Read the model definition and answer for the solid it produces. Units are mm, in the model's axes. A direction names the side the tool comes from. Give positions to 0.01 mm unless a question says otherwise; leave off trailing zeros. Write each loop counter-clockwise with the first axis right and the second up, starting at its lowest first coordinate (ties: lowest second). Pieces come first, ordered by that corner, then holes. Notation, with made-up numbers: (46, 41) -> (103, 41) arc R14 cw to (103, 52) -> close; hole circle Ø6 at (-2.75, 51). An arc over 180 degrees is marked (long way). Write item = value, one per line.
from build123d import *

# Parameters (mm, degrees)
CROQUIS1_W              = 240
CROQUIS1_H              = 260
SALIENTE_EXTRUIR1_DEPTH = 15
CROQUIS6_R              = 2.55
CORTAR_EXTRUIR3_DEPTH   = 178.552809046
CROQUIS7_R              = 5.5
CORTAR_EXTRUIR4_DEPTH   = 5
CROQUIS8_R              = 3.5
CORTAR_EXTRUIR5_DEPTH   = 178.552809046
CORTAR_EXTRUIR6_REACH   = 179.553
CROQUIS9_R              = 2.625
CROQUIS10_R             = 5.5
CORTAR_EXTRUIR7_DEPTH   = 5


with BuildPart() as part:
    # Croquis1 → Saliente-Extruir1 (new body)
    with BuildSketch(Plane(origin=(0, 0, 0), x_dir=(1, 0, 0), z_dir=(0, 1, 0))):
        Rectangle(CROQUIS1_W, CROQUIS1_H)
    extrude(amount=SALIENTE_EXTRUIR1_DEPTH)

    # Croquis6 → Cortar-Extruir3 (cut, through all)
    with BuildSketch(Plane.XZ):
        with Locations(Location((-45.5, -47.5, 0), (0, 0, 270))):
            Circle(CROQUIS6_R)
        with Locations(Location((-97.5, -47.5, 0), (0, 0, 270))):
            Circle(CROQUIS6_R)
        with Locations(Location((-97.5, 47.5, 0), (0, 0, 270))):
            Circle(CROQUIS6_R)
        with Locations(Location((-45.5, 47.5, 0), (0, 0, 270))):
            Circle(CROQUIS6_R)
        with Locations(Location((45.5, 47.5, 0), (0, 0, 270))):
            Circle(CROQUIS6_R)
        with Locations(Location((97.5, 47.5, 0), (0, 0, 270))):
            Circle(CROQUIS6_R)
        with Locations(Location((45.5, -47.5, 0), (0, 0, 270))):
            Circle(CROQUIS6_R)
        with Locations(Location((97.5, -47.5, 0), (0, 0, 270))):
            Circle(CROQUIS6_R)
    extrude(amount=-CORTAR_EXTRUIR3_DEPTH, mode=Mode.SUBTRACT)

    # Croquis7 → Cortar-Extruir4 (cut)
    with BuildSketch(Plane(origin=(0, 15, 0), x_dir=(1, 0, 0), z_dir=(0, 1, 0))):
        with Locations(Location((-97.5, 47.5, 0), (0, 0, 270))):
            Circle(CROQUIS7_R)
        with Locations(Location((-45.5, 47.5, 0), (0, 0, 270))):
            Circle(CROQUIS7_R)
        with Locations(Location((-97.5, -47.5, 0), (0, 0, 270))):
            Circle(CROQUIS7_R)
        with Locations(Location((-45.5, -47.5, 0), (0, 0, 270))):
            Circle(CROQUIS7_R)
        with Locations(Location((45.5, -47.5, 0), (0, 0, 270))):
            Circle(CROQUIS7_R)
        with Locations(Location((97.5, -47.5, 0), (0, 0, 270))):
            Circle(CROQUIS7_R)
        with Locations(Location((97.5, 47.5, 0), (0, 0, 270))):
            Circle(CROQUIS7_R)
        with Locations(Location((45.5, 47.5, 0), (0, 0, 270))):
            Circle(CROQUIS7_R)
    extrude(amount=-CORTAR_EXTRUIR4_DEPTH, mode=Mode.SUBTRACT)

    # Croquis8 → Cortar-Extruir5 (cut, through all)
    with BuildSketch(Plane(origin=(0, 15, 0), x_dir=(1, 0, 0), z_dir=(0, 1, 0))):
        with Locations(Location((-100, 100, 0), (0, 0, 270))):
            Circle(CROQUIS8_R)
        with Locations(Location((-50, 100, 0), (0, 0, 270))):
            Circle(CROQUIS8_R)
        with Locations(Location((0, 100, 0), (0, 0, 270))):
            Circle(CROQUIS8_R)
        with Locations(Location((50, 100, 0), (0, 0, 270))):
            Circle(CROQUIS8_R)
        with Locations(Location((100, 100, 0), (0, 0, 270))):
            Circle(CROQUIS8_R)
        with Locations(Location((0, 50, 0), (0, 0, 270))):
            Circle(CROQUIS8_R)
        with Locations(Location((-50, 0, 0), (0, 0, 270))):
            Circle(CROQUIS8_R)
        with Locations(Location((50, 0, 0), (0, 0, 270))):
            Circle(CROQUIS8_R)
        with Locations(Location((100, 0, 0), (0, 0, 270))):
            Circle(CROQUIS8_R)
        with Locations(Location((0, -50, 0), (0, 0, 270))):
            Circle(CROQUIS8_R)
        with Locations(Location((-50, -100, 0), (0, 0, 270))):
            Circle(CROQUIS8_R)
        with Locations(Location((0, -100, 0), (0, 0, 270))):
            Circle(CROQUIS8_R)
        with Locations(Location((50, -100, 0), (0, 0, 270))):
            Circle(CROQUIS8_R)
        with Locations(Location((100, -100, 0), (0, 0, 270))):
            Circle(CROQUIS8_R)
        with Locations(Location((-100, 0, 0), (0, 0, 270))):
            Circle(CROQUIS8_R)
        with Locations(Location((-100, -100, 0), (0, 0, 270))):
            Circle(CROQUIS8_R)
    extrude(amount=-CORTAR_EXTRUIR5_DEPTH, mode=Mode.SUBTRACT)

    # Croquis9 → Cortar-Extruir6 (cut, up to next)
    with BuildSketch(Plane.XZ, mode=Mode.PRIVATE) as cortar_extruir6_sk1:
        with Locations(Location((23.5, 30, 0), (0, 0, 270))):
            Circle(CROQUIS9_R)
    cortar_extruir6_tool1 = extrude(cortar_extruir6_sk1.sketch, amount=-CORTAR_EXTRUIR6_REACH, mode=Mode.PRIVATE) & part.part
    # Croquis9 → Cortar-Extruir6 (cut, up to next)
    with BuildSketch(Plane.XZ, mode=Mode.PRIVATE) as cortar_extruir6_sk2:
        with Locations(Location((-23.5, 30, 0), (0, 0, 270))):
            Circle(CROQUIS9_R)
    cortar_extruir6_tool2 = extrude(cortar_extruir6_sk2.sketch, amount=-CORTAR_EXTRUIR6_REACH, mode=Mode.PRIVATE) & part.part
    # Croquis9 → Cortar-Extruir6 (cut, up to next)
    with BuildSketch(Plane.XZ, mode=Mode.PRIVATE) as cortar_extruir6_sk3:
        with Locations(Location((-23.5, -30, 0), (0, 0, 270))):
            Circle(CROQUIS9_R)
    cortar_extruir6_tool3 = extrude(cortar_extruir6_sk3.sketch, amount=-CORTAR_EXTRUIR6_REACH, mode=Mode.PRIVATE) & part.part
    # Croquis9 → Cortar-Extruir6 (cut, up to next)
    with BuildSketch(Plane.XZ, mode=Mode.PRIVATE) as cortar_extruir6_sk4:
        with Locations(Location((23.5, -30, 0), (0, 0, 270))):
            Circle(CROQUIS9_R)
    cortar_extruir6_tool4 = extrude(cortar_extruir6_sk4.sketch, amount=-CORTAR_EXTRUIR6_REACH, mode=Mode.PRIVATE) & part.part
    add(cortar_extruir6_tool1.solids().sort_by_distance((23.5, 0, 30))[0], mode=Mode.SUBTRACT)
    add(cortar_extruir6_tool2.solids().sort_by_distance((-23.5, 0, 30))[0], mode=Mode.SUBTRACT)
    add(cortar_extruir6_tool3.solids().sort_by_distance((-23.5, 0, -30))[0], mode=Mode.SUBTRACT)
    add(cortar_extruir6_tool4.solids().sort_by_distance((23.5, 0, -30))[0], mode=Mode.SUBTRACT)

    # Croquis10 → Cortar-Extruir7 (cut)
    with BuildSketch(Plane(origin=(0, 15, 0), x_dir=(1, 0, 0), z_dir=(0, 1, 0))):
        with Locations(Location((-23.5, -30, 0), (0, 0, 270))):
            Circle(CROQUIS10_R)
        with Locations(Location((23.5, -30, 0), (0, 0, 270))):
            Circle(CROQUIS10_R)
        with Locations(Location((23.5, 30, 0), (0, 0, 270))):
            Circle(CROQUIS10_R)
        with Locations(Location((-23.5, 30, 0), (0, 0, 270))):
            Circle(CROQUIS10_R)
    extrude(amount=-CORTAR_EXTRUIR7_DEPTH, mode=Mode.SUBTRACT)


solid = part.part
(1) A tool of negligible diameter and unlimited length cuts with its end or side. For faces 1 (the cylindrical face through (27.22, 12.54, 25.95)), 2 (the cylindrical face through (-47.05, 7.6, 101.88)), from which of +Z, -Z, +X, -X, +Y, -Y can it reach the whole face along a straight path? Write none if from no direction.
Checks:
face_1 = +Y
face_2 = +Y, -Y
(2) The part is cut by section A-A on z = -100. Determine the outline of the cut face in (x, y).
Checks:
outline = (-120, 0) -> (-103.5, 0) -> (-103.5, 15) -> (-120, 15) -> close; (-96.5, 0) -> (-53.5, 0) -> (-53.5, 15) -> (-96.5, 15) -> close; (-46.5, 0) -> (-3.5, 0) -> (-3.5, 15) -> (-46.5, 15) -> close; (3.5, 0) -> (46.5, 0) -> (46.5, 15) -> (3.5, 15) -> close; (53.5, 0) -> (96.5, 0) -> (96.5, 15) -> (53.5, 15) -> close; (103.5, 0) -> (120, 0) -> (120, 15) -> (103.5, 15) -> close
(3) Consider L1, parallel to Z at x = 23, y = 6.5; L2, parallel to X at y = 6.25, z = 100; L3, parallel to X at y = 3.5, z = 30 (3 decimals). Determine where each line is inside the solid, lowest interval first.
Checks:
L1 = -130 to -32.58, -27.42 to 27.42, 32.58 to 130
L2 = -120 to -103.5, -96.5 to -53.5, -46.5 to -3.5, 3.5 to 46.5, 53.5 to 96.5, 103.5 to 120
L3 = -120 to -26.125, -20.875 to 20.875, 26.125 to 120
(4) For a pull along Z with two mould halves and no side action, classify faces 3 (the cylindrical face through (96.583, 7.605, -0.759)), 4 (the flat face through (-2, 7, 130)), 5 (the flat face through (120, 7, 2)), 6 (the cylindrical face through (27.22, 12.54, -34.05)) as released by +Z, released by -Z, zero draft, split by the parting line, or undercut.
Checks:
face_3 = undercut
face_4 = released by +Z
face_5 = zero draft
face_6 = undercut
(5) Given P1, Ø9, axis at x = 23.5, z = -30, coming from the +Y side, flat-ended and moving along its own axis, determine where the tip first touches the part or whether it passes through.
Checks:
P1 = 10
